from build123d import *

# Parameters (mm, degrees)
BOSS_EXTRUDE2_DEPTH = 50
SKETCH3_R           = 1.5
CUT_EXTRUDE1_DEPTH  = 50


with BuildPart() as part:
    # Sketch1 → Boss-Extrude2 (new body)
    with BuildSketch(Plane.XY):
        with BuildLine():
            Line((-7.452830189, -1.235849057), (-7.452830189, -11.235849057))
            Line((-7.452830189, -11.235849057), (12.547169811, -11.235849057))
            Line((12.547169811, -11.235849057), (12.547169811, 78.864150943))
            ThreePointArc((12.547169811, 78.864150943), (21.304677054, 100.006643701), (42.447169811, 108.764150943))
            Line((42.447169811, 108.764150943), (42.647169811, 108.764150943))
            ThreePointArc((42.647169811, 108.764150943), (63.789662569, 100.006643701), (72.547169811, 78.864150943))
            Line((72.547169811, 78.864150943), (72.547169811, -11.235849057))
            Line((72.547169811, -11.235849057), (92.547169811, -11.235849057))
            Line((92.547169811, -11.235849057), (92.547169811, -1.235849057))
            Line((92.547169811, -1.235849057), (82.547169811, -1.235849057))
            Line((82.547169811, -1.235849057), (82.547169811, 77.704131501))
            ThreePointArc((82.547169811, 77.704131501), (70.890019703, 105.846981392), (42.747169811, 117.504131501))
            Line((42.747169811, 117.504131501), (42.347169811, 117.504131501))
            ThreePointArc((42.347169811, 117.504131501), (14.20431992, 105.846981392), (2.547169811, 77.704131501))
            Line((2.547169811, 77.704131501), (2.547169811, -1.235849057))
            Line((2.547169811, -1.235849057), (-7.452830189, -1.235849057))
        make_face()
    extrude(amount=BOSS_EXTRUDE2_DEPTH)

    # Sketch3 → Cut-Extrude1 (cut)
    with BuildSketch(Plane(origin=(0, -1.235849057, 0), x_dir=(1, 0, 0), z_dir=(0, 1, 0))):
        with Locations(Location((-2.452830189, -40, 0), (0, 0, 270))):
            Circle(SKETCH3_R)
        with Locations(Location((-2.452830189, -10, 0), (0, 0, 270))):
            Circle(SKETCH3_R)
        with Locations(Location((87.547169811, -10, 0), (0, 0, 270))):
            Circle(SKETCH3_R)
        with Locations(Location((87.547169811, -40, 0), (0, 0, 270))):
            Circle(SKETCH3_R)
    extrude(amount=-CUT_EXTRUDE1_DEPTH, mode=Mode.SUBTRACT)


solid = part.part
Verification items for the finished model (mm, model axes). A direction names the side the tool comes from. Give positions to 0.01 mm unless a question says otherwise; leave off trailing zeros. Write each loop counter-clockwise with the first axis right and the second up, starting at its lowest first coordinate (ties: lowest second). Pieces come first, ordered by that corner, then holes. Notation, with made-up numbers: M -2.5,70.5 L 36.5,70.5 A23 ccw 36.5,79.5 Z; hole C 29,-16 d9. An arc over 180 degrees is marked long. Write item = value, one per line.
(1) Sectioned sample at C-C (y = 95.5). Record the cut outline in (x, z), then the cut area to 3 significant figures.
Found:
outline = M 6.75,0 L 17.6,0 L 17.6,50 L 6.75,50 Z; M 67.49,0 L 78.35,0 L 78.35,50 L 67.49,50 Z
area = 1,090 mm2
(2) Sectioned sample at D-D (x = 81). Record the cut outline in (y, z), then the cut area to 3 significant figures.
Found:
outline = M -11.24,0 L 88.69,0 L 88.69,50 L -11.24,50 Z
area = 5,000 mm2
(3) Go/stop test with flat-tipped pins: pin 1 Ø6 at (x, z) = (8, 18) entering from +Y; pin 2 Ø1.5 at (x, z) = (19, 7.5) entering from +Y; pin 3 Ø5 at (x, z) = (64, 25.5) entering from +Y; pin 4 Ø1.8 at (x, z) = (-2.45, 40) entering from -Y. Record where each tip stops, or that it passes through.
Found:
pin_1 = 102.23
pin_2 = 110.47
pin_3 = 112.81
pin_4 = through
(4) Sectioned sample at A-A (z = 40). Record the cut outline in (x, y).
Found:
outline = M -7.45,-11.24 L -3.95,-11.24 L -3.95,-1.24 L -7.45,-1.24 Z; M -0.95,-11.24 L 12.55,-11.24 L 12.55,78.86 A29.9 cw 42.45,108.76 L 42.65,108.76 A29.9 cw 72.55,78.86 L 72.55,-11.24 L 86.05,-11.24 L 86.05,-1.24 L 82.55,-1.24 L 82.55,77.7 A39.8 ccw 42.75,117.5 L 42.35,117.5 A39.8 ccw 2.55,77.7 L 2.55,-1.24 L -0.95,-1.24 Z; M 89.05,-11.24 L 92.55,-11.24 L 92.55,-1.24 L 89.05,-1.24 Z
(5) Draft check along X on faces 1 (the face through (2, -11.236, 25)), 2 (the face through (14.515, 106.155, 24.65)), 3 (the face through (72.547, 34, 25)). Enter one of: released by +X, released by -X, zero draft, split by the parting line, or undercut.
Found:
face_1 = zero draft
face_2 = released by -X
face_3 = undercut
(6) Material ranges on line 1 (X direction, y = -5.75, z = 10); line 2 (X direction, y = 11, z = 27.5), recorded low to high.
Found:
line_1 = -7.45 to -3.95, -0.95 to 12.55, 72.55 to 86.05, 89.05 to 92.55
line_2 = 2.55 to 12.55, 72.55 to 82.55
(7) Sectioned sample at B-B (y = 52). Record the cut outline in (x, z), then the cut area to 3 significant figures.
Found:
outline = M 2.55,0 L 12.55,0 L 12.55,50 L 2.55,50 Z; M 72.55,0 L 82.55,0 L 82.55,50 L 72.55,50 Z
area = 1,000 mm2
(8) Access from +Z, -Z, +X, -X, +Y, -Y to the whole of each face (thin tool, end or side, straight path). Record for faces 4 (the face through (86.216, -6.166, 10.692)), 5 (the face through (2.547, 39, 25)), 6 (the face through (82.547, 38, 25)), 7 (the face through (12.547, 33, 25)).
Found:
face_4 = +Y, -Y
face_5 = +Z, -Z, -X, +Y
face_6 = +Z, -Z, +X, +Y
face_7 = +Z, -Z, -Y
